from build123d import *

# Parameters (mm, degrees)
SKETCH_2_W          = 123.80594
SKETCH_2_H          = 24.590071156
EXTRUDE_2_DEPTH     = 3
SKETCH_3_R          = 3.5
SKETCH_3_R_2        = 2.5
EXTRUDE_3_DEPTH     = 9
EXTRUDE_4_DEPTH     = 9
SKETCH_7_W          = 100.499997397
SKETCH_7_H          = 7
CUT_EXTRUDE_1_DEPTH = 9
SKETCH_8_R          = 2.5
CUT_EXTRUDE_2_DEPTH = 153.544398733
FILLET_1_R          = 2
CUT_EXTRUDE_START   = -9
SKETCH_9_R          = 2.5
CUT_EXTRUDE_3_DEPTH = 9


# Read off the part's stored shape, not the designer's step: 凸台-拉伸4
with BuildPart() as part:
    # 草图2 → 凸台-拉伸2 (new body)
    with BuildSketch(Plane(origin=(0, 0, 0), x_dir=(1, 0, 0), z_dir=(0, 1, 0))):
        with Locations((61.90297, 12.720846688)):
            Rectangle(SKETCH_2_W, SKETCH_2_H)
        Polygon((149.999997397, 8.59581111), (123.80594, 0.42581111), (123.80594, 25.015882266), (149.999997397, 16.845882266), align=None)
    extrude(amount=EXTRUDE_2_DEPTH)

    # 草图3 → 凸台-拉伸3 (add)
    # profile 1 of 4: a face of its own
    with BuildSketch(Plane(origin=(0, 3, 0), x_dir=(1, 0, 0), z_dir=(0, 1, 0))):
        with Locations(Location((5.5, 19.515882266, 0), (0, 0, 270))):
            Circle(SKETCH_3_R)
        with Locations(Location((5.5, 19.515882266, 0), (0, 0, 270))):
            Circle(SKETCH_3_R_2, mode=Mode.SUBTRACT)
    # profile 2 of 4: a face of its own
    with BuildSketch(Plane(origin=(0, 3, 0), x_dir=(1, 0, 0), z_dir=(0, 1, 0))):
        with Locations(Location((19.5, 19.515882266, 0), (0, 0, 270))):
            Circle(SKETCH_3_R)
        with Locations(Location((19.5, 19.515882266, 0), (0, 0, 270))):
            Circle(SKETCH_3_R_2, mode=Mode.SUBTRACT)
    # profile 3 of 4: a face of its own
    with BuildSketch(Plane(origin=(0, 3, 0), x_dir=(1, 0, 0), z_dir=(0, 1, 0))):
        with Locations(Location((19.5, 5.515882266, 0), (0, 0, 270))):
            Circle(SKETCH_3_R)
        with Locations(Location((19.5, 5.515882266, 0), (0, 0, 270))):
            Circle(SKETCH_3_R_2, mode=Mode.SUBTRACT)
    # profile 4 of 4: a face of its own
    with BuildSketch(Plane(origin=(0, 3, 0), x_dir=(1, 0, 0), z_dir=(0, 1, 0))):
        with Locations(Location((5.5, 5.515882266, 0), (0, 0, 270))):
            Circle(SKETCH_3_R)
        with Locations(Location((5.5, 5.515882266, 0), (0, 0, 270))):
            Circle(SKETCH_3_R_2, mode=Mode.SUBTRACT)
    extrude(amount=EXTRUDE_3_DEPTH)

    # 凸台-拉伸4 outline → 凸台-拉伸4 (add)
    with BuildSketch(Plane(origin=(0, 3, 0), x_dir=(1, 0, 0), z_dir=(0, 1, 0))):
        with BuildLine():
            Line((19.525916812, 2.015978222), (130.218193953, 2.42581111))
            Line((130.218193953, 2.42581111), (149.999997397, 8.59581111))
            Line((149.999997397, 8.59581111), (149.999997397, 16.845882266))
            Line((149.999997397, 16.845882266), (130.218193953, 23.015882266))
            Line((130.218193953, 23.015882266), (19.5, 23.015882266))
            ThreePointArc((19.5, 23.015882266), (23, 19.515882266), (19.5, 16.015882266))
            Line((19.5, 16.015882266), (19.5, 9.015882266))
            ThreePointArc((19.5, 9.015882266), (22.999976011, 5.528840761), (19.525916812, 2.015978222))
        make_face()
    extrude(amount=EXTRUDE_4_DEPTH)

    # 草图7 → 切除-拉伸1 (cut)
    with BuildSketch(Plane(origin=(0, 12, 0), x_dir=(1, 0, 0), z_dir=(0, 1, 0))):
        with Locations((79.749998699, 12.515882266)):
            Rectangle(SKETCH_7_W, SKETCH_7_H)
    extrude(amount=-CUT_EXTRUDE_1_DEPTH, mode=Mode.SUBTRACT)

    # 草图8 → 切除-拉伸2 (cut, through all)
    with BuildSketch(Plane.XZ):
        with Locations(Location((143.499997397, -12.515882266, 0), (0, 0, 270))):
            Circle(SKETCH_8_R)
    extrude(amount=-CUT_EXTRUDE_2_DEPTH, mode=Mode.SUBTRACT)

    # 圆角1
    fillet_1_edges = [part.edges().sort_by_distance(p)[0] for p in [
        (19.5, 7.5, -16.015882266),
        (19.5, 7.5, -9.015882266),
        (29.5, 7.5, -9.015882266),
        (29.5, 7.5, -16.015882266),
        (129.999997397, 7.5, -16.015882266),
        (129.999997397, 7.5, -9.015882266),
    ]]
    fillet(fillet_1_edges, radius=FILLET_1_R)

    # 草图9 → 切除-拉伸3 (cut)
    with BuildSketch(Plane(origin=(0, 3, 0), x_dir=(1, 0, 0), z_dir=(0, 1, 0)).offset(CUT_EXTRUDE_START)):
        with Locations(Location((5.5, 5.515882266, 0), (0, 0, 270))):
            Circle(SKETCH_9_R)
        with Locations(Location((19.5, 5.515882266, 0), (0, 0, 270))):
            Circle(SKETCH_9_R)
        with Locations(Location((19.5, 19.515882266, 0), (0, 0, 270))):
            Circle(SKETCH_9_R)
        with Locations(Location((5.5, 19.515882266, 0), (0, 0, 270))):
            Circle(SKETCH_9_R)
    extrude(amount=CUT_EXTRUDE_3_DEPTH, mode=Mode.SUBTRACT)


solid = part.part
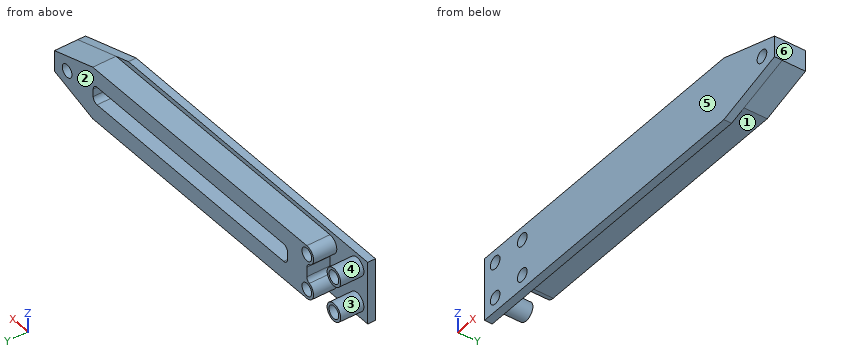
Verification items for the finished model (mm, model axes). Face numbers are marked on the shaded views. A direction names the side the tool comes from. Coordinates: 2 decimals unless noted, no trailing zeros. Order: outer loops, then holes, each group sorted by start corner. A loop starts at its lowest first (then second) coordinate and runs counter-clockwise, first axis right, second up. Notation, with made-up numbers: M 2,-13.5 L 40,-13.5 A25 cw 40,18.5 Z; hole C 31,50 d3. An arc over 180 degrees is marked long. One line per item, written item: value. Start each with the question number.
Item 1: Scan lines: probe 1 along Z at (x, y) = (123, 9.25); probe 2 along Y at (x, z) = (74, -10); probe 3 along X at (y, z) = (1, -13.25). Record each from-to range of solid material in increasing order.
Item 2: Access from +Z, -Z, +X, -X, +Y, -Y to the whole of each face (thin tool, end or side, straight path). Record for the marked faces 1, 2 and 3.
Item 3: Sectioned sample at A-A (x = 5.5). Enter the section's corners in (y, z).
Item 4: Sectioned sample at D-D (x = 25). Enter the section's corners in (y, z), then the cut area to 3 significant figures.
Item 5: Mould release check, pull along X, two halves, no side actions. Record for the marked faces 4, 5 and 6: released by +X, released by -X, zero draft, split by the parting line, or undercut.
Item 6: Sectioned sample at B-B (z = -5.75). Enter the section's corners in (x, y), then the cut area to 3 significant figures.
Item 7: Sectioned sample at C-C (x = 97). Enter the section's corners in (y, z), then the cut area to 3 significant figures.
Item 8: Gauge pin test, flat ends, axial feed: pin 1 (4.5 mm diameter, centred on x = 93.5, y = 8, fed in from -Z); pin 2 (1.9 mm diameter, centred on y = 6, z = -11.5, fed in from -X); pin 3 (6 mm diameter, centred on y = 7.5, z = -8.5, fed in from -X); pin 4 (3 mm diameter, centred on x = 143.5, z = -12.52, fed in from +Y). Record the tip position at first contact, or that the pin passes through.
Conclusion:
1. probe 1: z = -23.02 to -16.02, -9.02 to -2.4
1. probe 2: y = 0 to 3
1. probe 3: x = 0 to 141.11, 145.89 to 150
2. face 1: -Z, +X, -X, +Y
2. face 2: +Z, -Z, +X, -X, +Y
2. face 3: +Y
3. outline: M 0,-25.02 L 3,-25.02 L 3,-23.02 L 12,-23.02 L 12,-22.02 L 0,-22.02 Z; M 0,-17.02 L 12,-17.02 L 12,-16.02 L 3,-16.02 L 3,-9.02 L 12,-9.02 L 12,-8.02 L 0,-8.02 Z; M 0,-3.02 L 12,-3.02 L 12,-2.02 L 3,-2.02 L 3,-0.43 L 0,-0.43 Z
4. outline: M 0,-25.02 L 3,-25.02 L 3,-23.02 L 12,-23.02 L 12,-2.04 L 3,-2.04 L 3,-0.43 L 0,-0.43 Z
4. area: 263 mm^2
5. face 4: undercut
5. face 5: zero draft
5. face 6: released by +X
6. outline: M 0,0 L 3.01,0 L 3.01,12 L 2.01,12 L 2.01,3 L 0,3 Z; M 7.99,0 L 17.01,0 L 17.01,12 L 16.01,12 L 16.01,3 L 8.99,3 L 8.99,12 L 7.99,12 Z; M 21.99,0 L 140.88,0 L 140.88,12 L 21.99,12 Z
6. area: 1,490 mm^2
7. outline: M 0,-25.02 L 3,-25.02 L 3,-23.02 L 12,-23.02 L 12,-16.02 L 3,-16.02 L 3,-9.02 L 12,-9.02 L 12,-2.3 L 3,-2.3 L 3,-0.43 L 0,-0.43 Z
7. area: 197 mm^2
8. pin 1: stops at z = -23.02
8. pin 2: stops at x = 19.5
8. pin 3: stops at x = 2
8. pin 4: passes through
